Geometry check sheet. Reference: the model listing, model coordinates, mm. A direction names the side the tool comes from. Round coordinates to 2 decimals unless told otherwise and drop trailing zeros. Order: outer loops, then holes, each group sorted by start corner. A loop starts at its lowest first (then second) coordinate and runs counter-clockwise, first axis right, second up. Notation, with made-up numbers: (-18.75, 7.5) - (35.25, 7.5) arc R27 cw to (35.25, 26.5) - close; hole circle Ø8 at (9.5, 36.25). An arc over 180 degrees is marked (long way). One line per question, with ' | ' between items. Start each with the question number.
Q1. Gauge pin test, flat ends, axial feed: P1, Ø9.5, axis at x = 14, y = 3, coming from the -Z side; P2, Ø12.5, axis at x = 16, z = -9.4, coming from the -Y side (3 decimals); P3, Ø6, axis at x = 14, y = -2.5, coming from the +Z side. Record the tip position at first contact, or that the pin passes through.
Q2. Tool access check on faces 4 (the face through (3.6, 9.07, -14.09)), 5 (the face through (3.6, 9.07, 15.16)), 6 (the face through (1.57, -12.27, -24.95)), 7 (the face through (2, -2, 25.4)), 8 (the face through (14.22, -1.655, 0.043)). Record the directions out of +Z, -Z, +X, -X, +Y, -Y that give a thin tool (end or side, any length) a straight path to the whole face; none if there is none.
Q3. Sectioned sample at B-B, the plane z = 12.7. Enter the section's corners in (x, y) (3 decimals).
Q4. Sectioned sample at C-C, the plane x = 12.5. Enter the section's corners in (y, z) (1 decimal).
Q5. Sectioned sample at A-A, the plane y = 0. Enter the section's corners in (x, z) (1 decimal).
Q6. Material ranges on line 1 along X through (y, z) = (11.05, -9.4); line 2 along Y through (x, z) = (2, -12); line 3 along X through (y, z) = (4, -11.5) (3 decimals), recorded low to high.
Q7. Sectioned sample at D-D, the plane z = -12.7. Enter the section's corners in (x, y) (3 decimals), then the cut area to 3 significant figures.
Q8. Mould release check, pull along Z, two halves, no side actions. Record for faces 1 (the face through (31.55, 11.13, -24.97)), 2 (the face through (1.57, -12.25, 24.97)), 3 (the face through (1.57, 0.14, 9.53)): +Z half, -Z half, draft (parallel to the pull), parting line (faces both ways), or undercut.
```python
from build123d import *

# Parameters (mm, degrees)
SKETCH2_W           = 50.8
SKETCH2_H           = 25.4
BOSS_EXTRUDE1_DEPTH = 3.175
SKETCH4_W           = 32
SKETCH4_H           = 63.5
BOSS_EXTRUDE2_DEPTH = 3.175
SKETCH6_R           = 3.175
CUT_EXTRUDE2_DEPTH  = 3.175
BOSS_EXTRUDE3_DEPTH = 1.5875
SKETCH8_R           = 4.85
CUT_EXTRUDE3_DEPTH  = 10
FILLET3_R           = 1.5


with BuildPart() as part:
    # Sketch2 → Boss-Extrude1 (new body)
    with BuildSketch(Plane(origin=(0, 0, 0), x_dir=(0, 0, -1), z_dir=(1, 0, 0))):
        Rectangle(SKETCH2_W, SKETCH2_H)
    extrude(amount=BOSS_EXTRUDE1_DEPTH)

    # Sketch4 → Boss-Extrude2 (add)
    with BuildSketch(Plane(origin=(0, 12.7, 0), x_dir=(1, 0, 0), z_dir=(0, 1, 0))):
        with Locations((16, -6.35)):
            Rectangle(SKETCH4_W, SKETCH4_H)
    extrude(amount=-BOSS_EXTRUDE2_DEPTH)

    # Sketch6 → Cut-Extrude2 (cut)
    with BuildSketch(Plane.ZY):
        with Locations((-12.7, 0)):
            Circle(SKETCH6_R)
        with Locations((12.7, 0)):
            Circle(SKETCH6_R)
    extrude(amount=-CUT_EXTRUDE2_DEPTH, mode=Mode.SUBTRACT)

    # Sketch7 → Boss-Extrude3 (add, symmetric)
    with BuildSketch(Plane.XY):
        Polygon((3.175, -12.7), (25.4, 9.525), (3.175, 9.525), align=None)
    extrude(amount=BOSS_EXTRUDE3_DEPTH, both=True)

    # Sketch8 → Cut-Extrude3 (cut)
    with BuildSketch(Plane(origin=(0, 12.7, 0), x_dir=(1, 0, 0), z_dir=(0, 1, 0))):
        with Locations(Location((16, 9.4, 0), (0, 0, 270))):
            Circle(SKETCH8_R)
        with Locations(Location((16, -23.536231777, 0), (0, 0, 270))):
            Circle(SKETCH8_R)
    extrude(amount=-CUT_EXTRUDE3_DEPTH, mode=Mode.SUBTRACT)

    # Fillet3
    # the kernel refuses this fillet: 1.5 mm, written as the material it adds along each edge
    with BuildSketch(Plane(origin=(4.675, 8.025, 3.0875), x_dir=(0, 0, -1), z_dir=(-1, 0, 0))) as fillet3_piece_1_section:
        Polygon((0, 0), (FILLET3_R, 0), (FILLET3_R, -FILLET3_R), (0, -FILLET3_R), align=None)
    fillet3_piece_1 = extrude(amount=FILLET3_R, mode=Mode.PRIVATE)
    fillet3_piece_1 = fillet3_piece_1 - Plane(origin=(4.675, 8.025, 3.0875), x_dir=(0, -0.7071067811865475, 0.7071067811865475), z_dir=(-1, 0, 0)) * Sphere(FILLET3_R, mode=Mode.PRIVATE)
    add(fillet3_piece_1)
    with BuildSketch(Plane(origin=(4.675, 8.025, -3.0875), x_dir=(-1, 0, 0), z_dir=(0, 0, 1))) as fillet3_piece_2_section:
        Polygon((0, 0), (FILLET3_R, 0), (FILLET3_R, -FILLET3_R), (0, -FILLET3_R), align=None)
    fillet3_piece_2 = extrude(amount=FILLET3_R, mode=Mode.PRIVATE)
    fillet3_piece_2 = fillet3_piece_2 - Plane(origin=(4.675, 8.025, -3.0875), x_dir=(0.7071067811865475, -0.7071067811865475, 0), z_dir=(0, 0, 1)) * Sphere(FILLET3_R, mode=Mode.PRIVATE)
    add(fillet3_piece_2)
    with BuildSketch(Plane(origin=(3.175, 9.525, 25.4), x_dir=(0, -1, 0), z_dir=(-1, 0, 0))) as fillet3_piece_3:
        with BuildLine():
            CenterArc((FILLET3_R, FILLET3_R), FILLET3_R, 180, 90)
            Line((0, FILLET3_R), (0, 0))
            Line((0, 0), (FILLET3_R, 0))
        make_face()
    extrude(amount=3.175)
    with BuildSketch(Plane(origin=(3.175, 9.525, 25.4), x_dir=(0, -1, 0), z_dir=(0, 0, -1)), Plane(origin=(3.175, 9.525, -3.0875), x_dir=(0, -1, 0), z_dir=(0, 0, -1))) as fillet3_piece_4:
        with BuildLine():
            CenterArc((FILLET3_R, -FILLET3_R), FILLET3_R, 90, 90)
            Line((0, -FILLET3_R), (0, 0))
            Line((0, 0), (FILLET3_R, 0))
        make_face()
    extrude(amount=22.3125)
    with BuildSketch(Plane(origin=(29.15, 9.525, -1.5875), x_dir=(0, 0, -1), z_dir=(-1, 0, 0))) as fillet3_piece_5_section:
        with BuildLine():
            CenterArc((FILLET3_R, FILLET3_R), FILLET3_R, 180, 90)
            Line((0, FILLET3_R), (0, 0))
            Line((0, 0), (FILLET3_R, 0))
        make_face()
    fillet3_piece_5 = extrude(amount=24.475, mode=Mode.PRIVATE)
    fillet3_piece_5 = split(fillet3_piece_5, bisect_by=Plane(origin=(19.967902823, 4.092902823, -1.930123153), z_dir=(-0.707106781186549, 0.707106781186546, 0)), keep=Keep.TOP, mode=Mode.PRIVATE)
    add(fillet3_piece_5)
    with BuildSketch(Plane(origin=(25.4, 9.525, -1.5875), x_dir=(-0.7071067811865489, -0.7071067811865461, 0), z_dir=(0, 0, 1))) as fillet3_piece_6:
        with BuildLine():
            CenterArc((FILLET3_R * 0.414213562373, FILLET3_R), FILLET3_R, 225, 45)
            Line((-FILLET3_R * 0.292893218813, FILLET3_R * 0.292893218813), (0, 0))
            Line((0, 0), (FILLET3_R * 0.414213562373, 0))
        make_face()
    extrude(amount=3.175)
    with BuildSketch(Plane(origin=(3.175, 8.025, -1.5875), x_dir=(0, 0, -1), z_dir=(0, -1, 0))) as fillet3_piece_7_section:
        with BuildLine():
            CenterArc((FILLET3_R, FILLET3_R), FILLET3_R, 180, 90)
            Line((0, FILLET3_R), (0, 0))
            Line((0, 0), (FILLET3_R, 0))
        make_face()
    fillet3_piece_7 = extrude(amount=20.725, mode=Mode.PRIVATE)
    fillet3_piece_7 = split(fillet3_piece_7, bisect_by=Plane(origin=(8.60741784, -7.26758216, -1.930100054), z_dir=(-0.707106781186549, 0.707106781186546, 0)), keep=Keep.TOP, mode=Mode.PRIVATE)
    add(fillet3_piece_7)
    with BuildSketch(Plane(origin=(29.15, 9.525, 1.5875), x_dir=(0, 0, 1), z_dir=(-1, 0, 0))) as fillet3_piece_8_section:
        with BuildLine():
            CenterArc((FILLET3_R, -FILLET3_R), FILLET3_R, 90, 90)
            Line((0, -FILLET3_R), (0, 0))
            Line((0, 0), (FILLET3_R, 0))
        make_face()
    fillet3_piece_8 = extrude(amount=24.475, mode=Mode.PRIVATE)
    fillet3_piece_8 = split(fillet3_piece_8, bisect_by=Plane(origin=(19.967902823, 4.092902823, 1.930123153), z_dir=(-0.707106781186549, 0.707106781186546, 0)), keep=Keep.TOP, mode=Mode.PRIVATE)
    add(fillet3_piece_8)
    with BuildSketch(Plane(origin=(3.175, 8.025, 1.5875), x_dir=(0, 0, 1), z_dir=(0, -1, 0))) as fillet3_piece_9_section:
        with BuildLine():
            CenterArc((FILLET3_R, -FILLET3_R), FILLET3_R, 90, 90)
            Line((0, -FILLET3_R), (0, 0))
            Line((0, 0), (FILLET3_R, 0))
        make_face()
    fillet3_piece_9 = extrude(amount=20.725, mode=Mode.PRIVATE)
    fillet3_piece_9 = split(fillet3_piece_9, bisect_by=Plane(origin=(8.60741784, -7.26758216, 1.930100054), z_dir=(-0.707106781186549, 0.707106781186546, 0)), keep=Keep.TOP, mode=Mode.PRIVATE)
    add(fillet3_piece_9)
    with BuildSketch(Plane(origin=(6.925, 9.525, 25.4), x_dir=(0, -1, 0), z_dir=(-1, 0, 0))) as fillet3_piece_10a_section:
        with BuildLine():
            CenterArc((FILLET3_R, FILLET3_R), FILLET3_R, 180, 90)
            Line((0, FILLET3_R), (0, 0))
            Line((0, 0), (FILLET3_R, 0))
        make_face()
    fillet3_piece_10a = extrude(amount=6.925, mode=Mode.PRIVATE)
    fillet3_piece_10a = split(fillet3_piece_10a, bisect_by=Plane(origin=(3.175, 9.185407329, 25.739592671), z_dir=(1, 0, 0)), keep=Keep.TOP, mode=Mode.PRIVATE)
    with BuildSketch(Plane(origin=(3.175, 9.525, 29.15), x_dir=(0, -1, 0), z_dir=(0, 0, -1))) as fillet3_piece_10b_section:
        with BuildLine():
            CenterArc((FILLET3_R, -FILLET3_R), FILLET3_R, 90, 90)
            Line((0, -FILLET3_R), (0, 0))
            Line((0, 0), (FILLET3_R, 0))
        make_face()
    fillet3_piece_10b = extrude(amount=26.0625, mode=Mode.PRIVATE)
    fillet3_piece_10b = split(fillet3_piece_10b, bisect_by=Plane(origin=(3.514592671, 9.185407329, 25.4), z_dir=(0, 0, 1)), keep=Keep.TOP, mode=Mode.PRIVATE)
    fillet3_piece_10 = fillet3_piece_10a & fillet3_piece_10b
    add(fillet3_piece_10)
    with BuildSketch(Plane(origin=(25.4, 9.525, -3.140800859), x_dir=(-0.7071067811865446, -0.7071067811865503, 0), z_dir=(0, 0, 1))) as fillet3_piece_11a_section:
        with BuildLine():
            CenterArc((FILLET3_R * 0.414213562373, FILLET3_R), FILLET3_R, 225, 45)
            Line((-FILLET3_R * 0.292893218813, FILLET3_R * 0.292893218813), (0, 0))
            Line((0, 0), (FILLET3_R * 0.414213562373, 0))
        make_face()
    fillet3_piece_11a = extrude(amount=4.728300859, mode=Mode.PRIVATE)
    fillet3_piece_11a = split(fillet3_piece_11a, bisect_by=Plane(origin=(25.438403899, 9.432284787, -1.5875), z_dir=(0, 0, -1)), keep=Keep.TOP, mode=Mode.PRIVATE)
    with BuildSketch(Plane(origin=(29.15, 9.525, -1.5875), x_dir=(0, 0, -1), z_dir=(-1, 0, 0))) as fillet3_piece_11b_section:
        with BuildLine():
            CenterArc((FILLET3_R, FILLET3_R), FILLET3_R, 180, 90)
            Line((0, FILLET3_R), (0, 0))
            Line((0, 0), (FILLET3_R, 0))
        make_face()
    fillet3_piece_11b = extrude(amount=24.475, mode=Mode.PRIVATE)
    fillet3_piece_11b = split(fillet3_piece_11b, bisect_by=Plane(origin=(26.063627713, 10.188627713, -1.91198662), z_dir=(0.707106781186549, -0.707106781186546, 0)), keep=Keep.TOP, mode=Mode.PRIVATE)
    fillet3_piece_11 = fillet3_piece_11a & fillet3_piece_11b
    add(fillet3_piece_11)
    with BuildSketch(Plane(origin=(25.4, 9.525, -1.5875), x_dir=(-0.7071067811865489, -0.7071067811865461, 0), z_dir=(0, 0, 1))) as fillet3_piece_12a_section:
        with BuildLine():
            CenterArc((FILLET3_R * 0.414213562373, FILLET3_R), FILLET3_R, 225, 45)
            Line((-FILLET3_R * 0.292893218813, FILLET3_R * 0.292893218813), (0, 0))
            Line((0, 0), (FILLET3_R * 0.414213562373, 0))
        make_face()
    fillet3_piece_12a = extrude(amount=4.728300859, mode=Mode.PRIVATE)
    fillet3_piece_12a = split(fillet3_piece_12a, bisect_by=Plane(origin=(25.438403899, 9.432284787, 1.5875), z_dir=(0, 0, 1)), keep=Keep.TOP, mode=Mode.PRIVATE)
    with BuildSketch(Plane(origin=(29.15, 9.525, 1.5875), x_dir=(0, 0, 1), z_dir=(-1, 0, 0))) as fillet3_piece_12b_section:
        with BuildLine():
            CenterArc((FILLET3_R, -FILLET3_R), FILLET3_R, 90, 90)
            Line((0, -FILLET3_R), (0, 0))
            Line((0, 0), (FILLET3_R, 0))
        make_face()
    fillet3_piece_12b = extrude(amount=24.475, mode=Mode.PRIVATE)
    fillet3_piece_12b = split(fillet3_piece_12b, bisect_by=Plane(origin=(26.063627713, 10.188627713, 1.91198662), z_dir=(0.707106781186549, -0.707106781186546, 0)), keep=Keep.TOP, mode=Mode.PRIVATE)
    fillet3_piece_12 = fillet3_piece_12a & fillet3_piece_12b
    add(fillet3_piece_12)
    # the kernel refuses this fillet: 1.5 mm, written as the material it takes off along each edge
    with BuildSketch(Plane(origin=(0, 16.45, 38.1), x_dir=(0, 0, -1), z_dir=(0, -1, 0)), Plane(origin=(32, 16.45, -25.4), x_dir=(0, 0, 1), z_dir=(0, -1, 0)), Plane(origin=(-3.75, -12.7, 25.4), x_dir=(0, 0, -1), z_dir=(1, 0, 0))) as fillet3_2_piece_1:
        with BuildLine():
            CenterArc((FILLET3_R, FILLET3_R), FILLET3_R, 180, 90)
            Line((0, FILLET3_R), (0, 0))
            Line((0, 0), (FILLET3_R, 0))
        make_face()
    extrude(amount=10.675, mode=Mode.SUBTRACT)
    with BuildSketch(Plane(origin=(32, 16.45, 38.1), x_dir=(0, 0, -1), z_dir=(0, -1, 0)), Plane(origin=(-3.75, -12.7, -25.4), x_dir=(0, 0, 1), z_dir=(1, 0, 0))) as fillet3_2_piece_2:
        with BuildLine():
            CenterArc((FILLET3_R, -FILLET3_R), FILLET3_R, 90, 90)
            Line((0, -FILLET3_R), (0, 0))
            Line((0, 0), (FILLET3_R, 0))
        make_face()
    extrude(amount=10.675, mode=Mode.SUBTRACT)


solid = part.part
```
Determined:
1) P1: stops at z = -1.59 | P2: stops at y = 9.525 | P3: stops at z = 1.59
2) face 4: -Z, +X, -Y | face 5: +Z, +X, -Y | face 6: -Z, +X, -X, -Y | face 7: +Z, +X, -X, -Y | face 8: +Z, -Z, +X, -Y
3) outline: (0, -12.7) - (3.175, -12.7) - (3.175, -3.175) - (0, -3.175) - close; (0, 3.175) - (3.175, 3.175) - (3.175, 8.025) arc R1.5 cw to (4.675, 9.525) - (32, 9.525) - (32, 12.7) - (0, 12.7) - close
4) outline: (-3.4, -1.6) - (8, -1.6) arc R1.5 cw to (9.5, -3.1) - (9.5, -6) - (12.7, -6) - (12.7, 20.2) - (9.5, 20.2) - (9.5, 3.1) arc R1.5 cw to (8, 1.6) - (-3.4, 1.6) - close; (9.5, -25.4) - (12.7, -25.4) - (12.7, -12.8) - (9.5, -12.8) - close; (9.5, 26.9) - (12.7, 26.9) - (12.7, 38.1) - (9.5, 38.1) - close
5) outline: (0, -25.4) - (3.2, -25.4) - (3.2, -15.9) - (0, -15.9) - close; (0, -9.5) - (3.2, -9.5) - (3.2, -3.1) arc R1.5 cw to (4.7, -1.6) - (15.9, -1.6) - (15.9, 1.6) - (4.7, 1.6) arc R1.5 cw to (3.2, 3.1) - (3.2, 9.5) - (0, 9.5) - close; (0, 15.9) - (3.2, 15.9) - (3.2, 25.4) - (0, 25.4) - close
6) line 1: x = 0 to 11.15, 20.85 to 32 | line 2: y = -12.7 to -3.1, 3.1 to 12.7 | line 3: x = 0 to 3.175
7) outline: (0, -12.7) - (3.175, -12.7) - (3.175, -3.175) - (0, -3.175) - close; (0, 3.175) - (3.175, 3.175) - (3.175, 8.025) arc R1.5 cw to (4.675, 9.525) - (12.446, 9.525) - (12.446, 12.7) - (0, 12.7) - close; (19.554, 9.525) - (32, 9.525) - (32, 12.7) - (19.554, 12.7) - close | area: 130 mm2
8) face 1: -Z half | face 2: +Z half | face 3: undercut
